from build123d import *

# Parameters (mm, degrees)
SKETCH1_W            = 20
SKETCH1_H            = 5
BOSS_EXTRUDE1_DEPTH  = 25.4
BOSS_EXTRUDE2_DEPTH  = 4
MIRROR2_COPY_1_DEPTH = 4


with BuildPart() as part:
    # Sketch1 → Boss-Extrude1 (new body)
    with BuildSketch(Plane.XY):
        with Locations((-10, 12.5)):
            Rectangle(SKETCH1_W, SKETCH1_H)
        Polygon((-20, 15), (-25, 15), (-25, -5), (-25, -10), (-20, -10), (-20, 10), align=None)
        with Locations((-35, -7.5)):
            Rectangle(SKETCH1_W, SKETCH1_H)
    boss_extrude1 = extrude(amount=BOSS_EXTRUDE1_DEPTH)

    # Sketch1_3 → Boss-Extrude2 (add)
    with BuildSketch(Plane.XY):
        Polygon((-25, -5), (-25, 15), (-45, -5), align=None)
    boss_extrude2 = extrude(amount=BOSS_EXTRUDE2_DEPTH)

    # Mirror1: Boss-Extrude2 across plane
    add(boss_extrude2.mirror(Plane.XY.offset(12.7)))

    # Sketch3 → M5 Clearance Hole1 (revolve, cut)
    with BuildSketch(Plane(origin=(-10, 15, 12.4), x_dir=(0, 0, 1), z_dir=(1, 0, 0))):
        Polygon((0, 0), (0, 13.652366702), (2.75, 12), (2.75, 0), align=None)
    m5_clearance_hole1 = revolve(axis=Axis((-10, 21.35, 12.4), (0, -1, 0)), mode=Mode.SUBTRACT)

    # Sketch5 → M5 Clearance Hole2 (revolve, cut)
    with BuildSketch(Plane(origin=(-25, 5, 12.4), x_dir=(0, 0, 1), z_dir=(0, 1, 0))):
        Polygon((0, 0), (0, 13.652366702), (2.75, 12), (2.75, 0), align=None)
    m5_clearance_hole2 = revolve(axis=Axis((-31.35, 5, 12.4), (1, 0, 0)), mode=Mode.SUBTRACT)

    # Sketch7 → 1_4 Clearance Hole1 (revolve, cut)
    with BuildSketch(Plane(origin=(-34.84, -5, 12.7), x_dir=(0, 0, 1), z_dir=(1, 0, 0))):
        Polygon((0, 0), (0, 14.029827343), (3.3782, 12), (3.3782, 0), align=None)
    f_1_4_clearance_hole1 = revolve(axis=Axis((-34.84, 1.35, 12.7), (0, -1, 0)), mode=Mode.SUBTRACT)

    # Mirror2: Boss-Extrude1, Boss-Extrude2, M5 Clearance Hole1, M5 Clearance Hole2, 1_4 Clearance Hole1 across plane
    add(boss_extrude1.mirror(Plane(origin=(0, 0, 0), x_dir=(0, 0, 1), z_dir=(1, 0, 0))))
    add(boss_extrude2.mirror(Plane(origin=(0, 0, 0), x_dir=(0, 0, 1), z_dir=(1, 0, 0))))
    add(m5_clearance_hole1.mirror(Plane(origin=(0, 0, 0), x_dir=(0, 0, 1), z_dir=(1, 0, 0))), mode=Mode.SUBTRACT)
    add(m5_clearance_hole2.mirror(Plane(origin=(0, 0, 0), x_dir=(0, 0, 1), z_dir=(1, 0, 0))), mode=Mode.SUBTRACT)
    add(f_1_4_clearance_hole1.mirror(Plane(origin=(0, 0, 0), x_dir=(0, 0, 1), z_dir=(1, 0, 0))), mode=Mode.SUBTRACT)

    # Mirror2 copy 1 sketch → Mirror2 copy 1 (add)
    with BuildSketch(Plane(origin=(0, 0, 25.4), x_dir=(-1, 0, 0), z_dir=(0, 0, -1))):
        Polygon((-25, -5), (-25, 15), (-45, -5), align=None)
    extrude(amount=MIRROR2_COPY_1_DEPTH)


solid = part.part
Can you work these out from the model? Positions are in its coordinate system, mm. A direction names the side the tool comes from. Round coordinates to 2 decimals unless told otherwise and drop trailing zeros. Write each loop counter-clockwise with the first axis right and the second up, starting at its lowest first coordinate (ties: lowest second). Pieces come first, ordered by that corner, then holes. Notation, with made-up numbers: (-11, 26) -> (13, 26) arc R15 ccw to (13, 31) -> close; hole circle Ø7 at (61.25, 67). An arc over 180 degrees is marked (long way). Use one line per item in the form item = value. Start each with the question number.
Q1. Which directions (+Z, -Z, +X, -X, +Y, -Y) give clear straight access to the entire face, cutting with the end or side of a thin tool? Please do faces 1 (the face through (-25, 7, 15)), 2 (the face through (0, 10, 13)), 3 (the face through (35.1, -5, 16.4)).
Q2. I'm going to push flat-ended pins straight in: P1, Ø5, axis at x = -7.5, z = 6, coming from the -Y side; P2, Ø8, axis at x = 14, y = 1, coming from the -Z side; P3, Ø11, axis at x = 34.84, z = 12.7, coming from the +Y side; P4, Ø14, axis at y = 4.5, z = 12, coming from the -X side. Where does each tip first touch, or does it pass through?
Q3. Imagine slicing it at B-B (x = -34.84). Please give me the cut outline in (y, z).
Q4. We'd pull the mould along Z, two halves only. Please class faces 4 (the face through (30, -10, 13)), 5 (the face through (-31, 1, 21.4)), 6 (the face through (1, 11, 0)): +Z half, -Z half, draft (parallel to the pull), parting line (faces both ways), or undercut.
Q5. Imagine slicing it at C-C (z = 2.5). Please give me the cut outline in (x, y), then the cut area to 3 significant figures.
Q6. If I drill on probe 1 along Z at (x, y) = (-10, 13.9); probe 2 along X at (y, z) = (11.75, 12.4); probe 3 along X at (y, z) = (-6, 17), over which ranges is the centre line in solid material (lowest first)? Write a range as [from, to].
Q7. Imagine slicing it at D-D (x = -10). Please give me the cut outline in (y, z).
Q8. Imagine slicing it at A-A (y = 5). Please give me the cut outline in (x, z), then the cut area to 3 significant figures.
Worked out:
q1.face_1 = -X, +Y
q1.face_2 = +Z, -Z, -Y
q1.face_3 = +X, +Y
q2.P1 = 10
q2.P2 = through
q2.P3 = -5
q2.P4 = -25
q3.outline = (-10, 0) -> (5.16, 0) -> (5.16, 4) -> (-5, 4) -> (-5, 9.32) -> (-10, 9.32) -> close; (-10, 16.08) -> (-5, 16.08) -> (-5, 21.4) -> (5.16, 21.4) -> (5.16, 25.4) -> (-10, 25.4) -> close
q4.face_4 = draft
q4.face_5 = undercut
q4.face_6 = -Z half
q5.outline = (-45, -10) -> (-20, -10) -> (-20, 10) -> (20, 10) -> (20, -10) -> (45, -10) -> (45, -5) -> (25, 15) -> (-25, 15) -> (-45, -5) -> close
q5.area = 1,050 mm^2
q6.probe_1 = [0, 9.65], [15.15, 25.4]
q6.probe_2 = [-25, -12.75], [-7.25, 7.25], [12.75, 25]
q6.probe_3 = [-45, -20], [20, 45]
q7.outline = (10, 0) -> (15, 0) -> (15, 9.65) -> (10, 9.65) -> close; (10, 15.15) -> (15, 15.15) -> (15, 25.4) -> (10, 25.4) -> close
q8.outline = (-35, 0) -> (-20, 0) -> (-20, 9.65) -> (-25, 9.65) -> (-25, 4) -> (-35, 4) -> close; (-35, 21.4) -> (-25, 21.4) -> (-25, 15.15) -> (-20, 15.15) -> (-20, 25.4) -> (-35, 25.4) -> close; (20, 0) -> (35, 0) -> (35, 4) -> (25, 4) -> (25, 9.65) -> (20, 9.65) -> close; (20, 15.15) -> (25, 15.15) -> (25, 21.4) -> (35, 21.4) -> (35, 25.4) -> (20, 25.4) -> close
q8.area = 359 mm^2
